For this review, take the finished solid that the model builds, in its own axes (mm). Face numbers are marked on the shaded views. Give positions to 0.01 mm unless a question says otherwise; leave off trailing zeros. Order: outer loops, then holes, each group sorted by start corner. A loop starts at its lowest first (then second) coordinate and runs counter-clockwise, first axis right, second up. Notation, with made-up numbers: (-6.5, -16) - (22.5, -16) arc R22 ccw to (22.5, 10) - close; hole circle Ø8 at (52.25, 82.25). An arc over 180 degrees is marked (long way). Use a Markdown table: item, result. Add a question column.
1) Mouldability with a two-part tool opening along Z and no side actions: class the marked faces 1 and 2 as released by +Z, released by -Z, zero draft, split by the parting line, or undercut.
2) We need section A-A on y = 0. Write out the cut boundary in (x, z) (3 decimals), then the cut area to 3 significant figures.
3) We need section C-C on z = -5. Write out the cut boundary in (x, y) (3 decimals), then the cut area to 3 significant figures.
4) We need section B-B on z = 0. Write out the cut boundary in (x, y) (3 decimals), then the cut area to 3 significant figures.
5) Wall thickness on L1, parallel to Z at x = 0, y = -47.5 (3 decimals); L2, parallel to Y at x = 2.5, z = -8; L3, parallel to Y at x = -1.9, z = 0 (3 decimals): over which ranges is each line inside the solid? List them lowest first.
6) Clearance check with a flat-ended pin moving along its axis: P1, Ø3, axis at y = -9.525, z = 0, coming from the +X side. State where the tip first meets the part, or that it passes through.
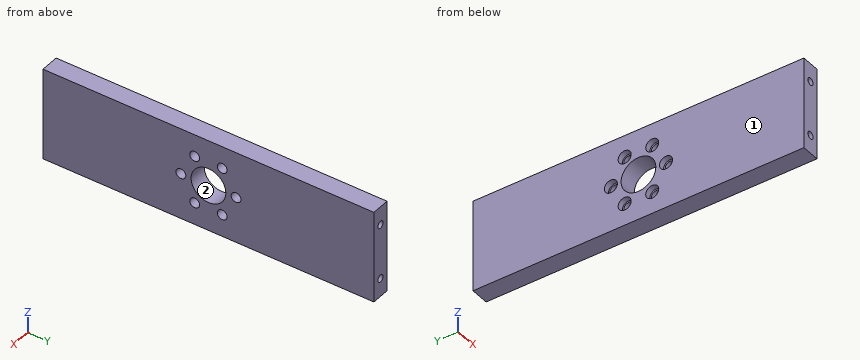
```python
from build123d import *

# Parameters (mm, degrees)
SKETCH1_W                      = 31.75
SKETCH1_H                      = 114.3
BOSS_EXTRUDE1_DEPTH            = 3.175
M3X0_5_TAPPED_HOLE1_AT_2_COUNT = 2
M3X0_5_TAPPED_HOLE1_AT_2_PITCH = 19.05
F_12_0MM_DOWEL_HOLE1_D         = 12
CBORE_FOR_M3_SHCS1_D           = 3.4
CBORE_FOR_M3_SHCS1_DEPTH       = 11.678536948
CBORE_FOR_M3_SHCS1_CBORE_D     = 4.5
CBORE_FOR_M3_SHCS1_CBORE_DEPTH = 2
CBORE_FOR_M3_SHCS1_TIP         = 1.021463052


with BuildPart() as part:
    # Sketch1 → Boss-Extrude1 (new, symmetric)
    with BuildSketch(Plane(origin=(0, 0, 0), x_dir=(0, 0, -1), z_dir=(1, 0, 0))):
        Rectangle(SKETCH1_W, SKETCH1_H)
    extrude(amount=BOSS_EXTRUDE1_DEPTH, both=True)

    # Sketch5 → M3x0.5 Tapped Hole1 (revolve, cut)
    with BuildSketch(Plane(origin=(0, 57.15, -9.525), x_dir=(0, 0, 1), z_dir=(1, 0, 0))):
        Polygon((0, 0), (0, 13.451075774), (1.25, 12.7), (1.25, 0), align=None)
    m3x0_5_tapped_hole1 = revolve(axis=Axis((0, 63.5, -9.525), (0, -1, 0)), mode=Mode.SUBTRACT)

    # M3x0.5 Tapped Hole1 at 2: M3x0.5 Tapped Hole1 ×2
    with Locations(*[(0, 0, i * M3X0_5_TAPPED_HOLE1_AT_2_PITCH) for i in range(1, M3X0_5_TAPPED_HOLE1_AT_2_COUNT)]):
        add(m3x0_5_tapped_hole1, mode=Mode.SUBTRACT)

    # Mirror1: M3x0.5 Tapped Hole1 across plane
    add(m3x0_5_tapped_hole1.mirror(Plane.ZX), mode=Mode.SUBTRACT)

    # Mirror1 copy 1 sketch → Mirror1 copy 1 (revolve, cut)
    with BuildSketch(Plane(origin=(0, -57.15, 9.525), x_dir=(0, 0, 1), z_dir=(1, 0, 0))):
        Polygon((0, 0), (0, -13.451075774), (1.25, -12.7), (1.25, 0), align=None)
    revolve(axis=Axis((0, -63.5, 9.525), (0, -1, 0)), mode=Mode.SUBTRACT)

    # Ø12.0mm Dowel Hole1 (through all)
    with Locations(Plane.ZY.offset(3.175)):
        with Locations((0, 0)):
            Hole(F_12_0MM_DOWEL_HOLE1_D / 2)

    # CBORE for M3 SHCS1
    with Locations(Plane.ZY.offset(3.175)):
        with Locations((8.248891971, -4.7625), (8.248891971, 4.7625), (0, 9.525), (-8.248891971, 4.7625), (-8.248891971, -4.7625), (0, -9.525)):
            CounterBoreHole(CBORE_FOR_M3_SHCS1_D / 2, CBORE_FOR_M3_SHCS1_CBORE_D / 2, CBORE_FOR_M3_SHCS1_CBORE_DEPTH, depth=CBORE_FOR_M3_SHCS1_DEPTH)
            with Locations((0, 0, -(CBORE_FOR_M3_SHCS1_DEPTH + CBORE_FOR_M3_SHCS1_TIP / 2))):  # 118° drill point
                Cone(0, CBORE_FOR_M3_SHCS1_D / 2, CBORE_FOR_M3_SHCS1_TIP, mode=Mode.SUBTRACT)


solid = part.part
```
Checked values:
| question | item | result |
|---|---|---|
| 1 | face 1 | zero draft |
| 1 | face 2 | undercut |
| 2 | outline | (-3.175, -15.875) - (3.175, -15.875) - (3.175, -6) - (-3.175, -6) - close; (-3.175, 6) - (3.175, 6) - (3.175, 15.875) - (-3.175, 15.875) - close |
| 2 | area | 125 mm² |
| 3 | outline | (-3.175, -57.15) - (3.175, -57.15) - (3.175, -3.317) - (-3.175, -3.317) - close; (-3.175, 3.317) - (3.175, 3.317) - (3.175, 57.15) - (-3.175, 57.15) - close |
| 3 | area | 684 mm² |
| 4 | outline | (-3.175, -57.15) - (3.175, -57.15) - (3.175, -11.225) - (-1.175, -11.225) - (-1.175, -11.775) - (-3.175, -11.775) - close; (-3.175, -7.275) - (-1.175, -7.275) - (-1.175, -7.825) - (3.175, -7.825) - (3.175, -6) - (-3.175, -6) - close; (-3.175, 6) - (3.175, 6) - (3.175, 7.825) - (-1.175, 7.825) - (-1.175, 7.275) - (-3.175, 7.275) - close; (-3.175, 11.775) - (-1.175, 11.775) - (-1.175, 11.225) - (3.175, 11.225) - (3.175, 57.15) - (-3.175, 57.15) - close |
| 4 | area | 602 mm² |
| 5 | L1 | -15.875 to -10.775, -8.275 to 8.275, 10.775 to 15.875 |
| 5 | L2 | -57.15 to -6.44, -3.08 to 3.08, 6.44 to 57.15 |
| 5 | L3 | -57.15 to -11.775, -7.275 to -6, 6 to 7.275, 11.775 to 57.15 |
| 6 | P1 | through |
